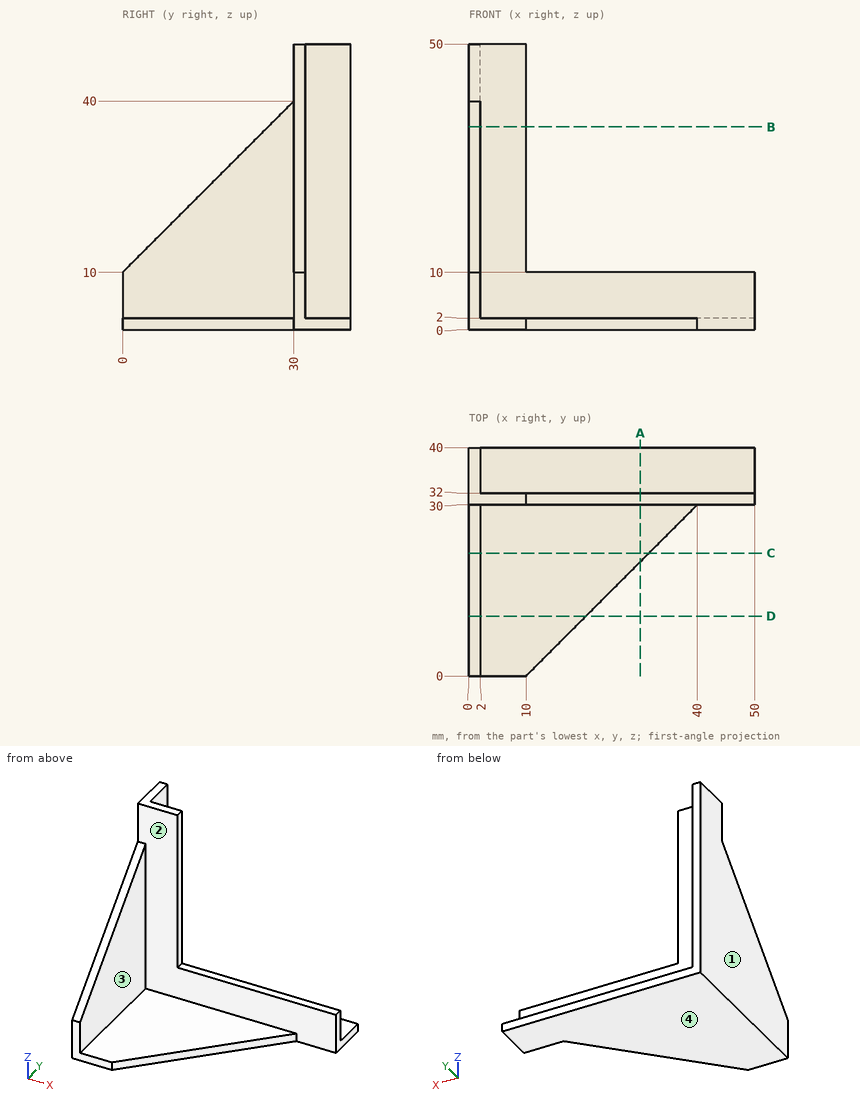
Study the drawing (mm; zero at the part's minimum x, y, z) and answer. A direction names the side the tool comes from. Coordinates: 2 decimals unless noted, no trailing zeros. Write each loop counter-clockwise with the first axis right and the second up, starting at its lowest first coordinate (ties: lowest second). Pieces come first, ordered by that corner, then holes. Notation, with made-up numbers: (-9.75, -13) -> (-3.75, -13) arc R11 cw to (-3.75, -5) -> close; hole circle Ø7 at (8.25, -5). An arc over 180 degrees is marked (long way). Write item = value, one per line.
(1) Section B-B on z = 35.5 is taken. Write down the section's boundary in (x, y), plus the area to 3 significant figures.
From the geometry:
outline = (0, 25.5) -> (2, 25.5) -> (2, 30) -> (10, 30) -> (10, 32) -> (2, 32) -> (2, 40) -> (0, 40) -> close
area = 45.0 mm2
(2) Section A-A on x = 30 is taken. Write down the section's boundary in (y, z).
From the geometry:
outline = (20, 0) -> (40, 0) -> (40, 2) -> (32, 2) -> (32, 10) -> (30, 10) -> (30, 2) -> (20, 2) -> close
(3) For a pull along Y with two mould halves and no side action, classify the marked faces 1 and 2 as +Y half, -Y half, draft (parallel to the pull), parting line (faces both ways), or undercut.
From the geometry:
face_1 = draft
face_2 = -Y half
(4) Given pin 1 Ø1.6 at (y, z) = (31.5, 28.5) entering from +X; pin 2 Ø1 at (x, z) = (7, 33.5) entering from -Y; pin 3 Ø1.6 at (x, y) = (36.5, 31.5) entering from +Z, each flat-ended and moving along its own axis, determine where each tip first touches the part or whether it passes through.
From the geometry:
pin_1 = 10
pin_2 = 30
pin_3 = 10
(5) Which of the six approach directions +Z, -Z, +X, -X, +Y, -Y give full straight-line access (tool end or side, diameter ignored) to the marked faces 3 and 4?
From the geometry:
face_3 = +Z, +X, -Y
face_4 = -Z, +X, -X, +Y, -Y
(6) Straight lines are drawn through the part: L1, parallel to X at y = 34.5, z = 33.5; L2, parallel to Y at x = 22, z = 6. For each, find the intervals that lie inside material, in ascending order. Write a range as from..to.
From the geometry:
L1 = 0..2
L2 = 30..32
(7) Section D-D on y = 10.5 is taken. Write down the section's boundary in (x, z), plus the area to 3 significant figures.
From the geometry:
outline = (0, 0) -> (20.5, 0) -> (20.5, 2) -> (2, 2) -> (2, 20.5) -> (0, 20.5) -> close
area = 78.0 mm2
(8) Section C-C on y = 21.5 is taken. Write down the section's boundary in (x, z), plus the area to 3 significant figures.
From the geometry:
outline = (0, 0) -> (31.5, 0) -> (31.5, 2) -> (2, 2) -> (2, 31.5) -> (0, 31.5) -> close
area = 122 mm2
